Here's how the part is built. I have some questions about the finished solid (model axes, mm). Face numbers are marked on the shaded views. A direction names the side the tool comes from. Round coordinates to 2 decimals unless told otherwise and drop trailing zeros. Write each loop counter-clockwise with the first axis right and the second up, starting at its lowest first coordinate (ties: lowest second). Pieces come first, ordered by that corner, then holes. Notation, with made-up numbers: (47.25, 73) -> (102.25, 73) arc R20 ccw to (102.25, 111) -> close; hole circle Ø3 at (46.5, 12). An arc over 180 degrees is marked (long way). Answer in a Markdown table with one row per item.
from build123d import *

# Parameters (mm, degrees)
SKETCH1_W           = 300
SKETCH1_H           = 56
BOSS_EXTRUDE1_DEPTH = 56
FILLET1_R           = 5
SKETCH2_R           = 27
SKETCH2_W           = 42
SKETCH2_H           = 2
SKETCH2_W_2         = 5
SKETCH2_H_2         = 5
CUT_EXTRUDE1_DEPTH  = 50
SKETCH3_W           = 69.790407192
SKETCH3_H           = 41
CUT_EXTRUDE2_DEPTH  = 25


with BuildPart() as part:
    # Sketch1 → Boss-Extrude1 (new body)
    with BuildSketch(Plane.XY):
        Rectangle(SKETCH1_W, SKETCH1_H)
    extrude(amount=BOSS_EXTRUDE1_DEPTH)

    # Fillet1
    fillet1_edges = [part.edges().sort_by_distance(p)[0] for p in [
        (-150, 0, 0),
        (0, 28, 0),
        (150, 0, 0),
        (-150, 28, 28),
        (150, 28, 28),
    ]]
    fillet(fillet1_edges, radius=FILLET1_R)

    # Sketch2 → Cut-Extrude1 (cut)
    with BuildSketch(Plane.XY.offset(56)):
        with Locations((-71.095356244, 0)):
            Circle(SKETCH2_R)
        with Locations((72.182261243, 0)):
            Rectangle(SKETCH2_W, SKETCH2_H)
        with Locations((110.682261243, 0)):
            Rectangle(SKETCH2_W_2, SKETCH2_H_2)
    extrude(amount=-CUT_EXTRUDE1_DEPTH, mode=Mode.SUBTRACT)

    # Sketch3 → Cut-Extrude2 (cut)
    with BuildSketch(Plane(origin=(0, 28, 0), x_dir=(1, 0, 0), z_dir=(0, 1, 0))):
        with Locations((80.104796404, -30.5)):
            Rectangle(SKETCH3_W, SKETCH3_H)
    extrude(amount=-CUT_EXTRUDE2_DEPTH, mode=Mode.SUBTRACT)


solid = part.part
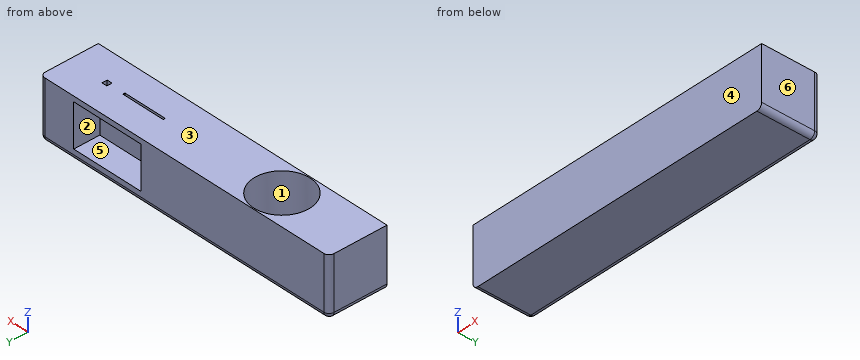
1) I want a section at C-C, the plane x = -92. List the corners of the cut face in (y, z) for me, and give its area (3 significant figures).
Response:
| item | result |
|---|---|
| outline | (-28, 0) -> (23, 0) arc R5 ccw to (28, 5) -> (28, 56) -> (17.09, 56) -> (17.09, 6) -> (-17.09, 6) -> (-17.09, 56) -> (-28, 56) -> close |
| area | 1,420 mm^2 |
2) We'd pull the mould along X, two halves only. Please class the marked faces 4, 5 and 6: +X half, -X half, draft (parallel to the pull), parting line (faces both ways), or undercut.
Response:
| item | result |
|---|---|
| face 4 | draft |
| face 5 | undercut |
| face 6 | +X half |
3) I want a section at D-D, the plane y = 7. List the corners of the cut face in (x, z) for me, and give its area (3 significant figures).
Response:
| item | result |
|---|---|
| outline | (-150, 5) arc R5 ccw to (-145, 0) -> (145, 0) arc R5 ccw to (150, 5) -> (150, 56) -> (-45.02, 56) -> (-45.02, 6) -> (-97.17, 6) -> (-97.17, 56) -> (-150, 56) -> close; hole (45.21, 10) -> (115, 10) -> (115, 51) -> (45.21, 51) -> close |
| area | 11,300 mm^2 |
4) I need wall thicknesses on line 1 (Y direction, x = 61.5, z = 47); line 2 (Z direction, x = -58, y = -15.5); line 3 (Y direction, x = -78, z = 53). Which ranges of each line are inside material? Lowest first, please. Write a range as [from, to].
Response:
| item | result |
|---|---|
| line 1 | y = [-28, -1], [1, 3] |
| line 2 | z = [0, 6] |
| line 3 | y = [-28, -26.1], [26.1, 28] |
5) I want a section at B-B, the plane y = -11. List the corners of the cut face in (x, z) for me, and give its area (3 significant figures).
Response:
| item | result |
|---|---|
| outline | (-150, 5) arc R5 ccw to (-145, 0) -> (145, 0) arc R5 ccw to (150, 5) -> (150, 56) -> (-46.44, 56) -> (-46.44, 6) -> (-95.75, 6) -> (-95.75, 56) -> (-150, 56) -> close |
| area | 14,300 mm^2 |
6) I want a section at A-A, the plane z = 53.5. List the corners of the cut face in (x, y) for me, and give its area (3 significant figures).
Response:
| item | result |
|---|---|
| outline | (-150, -28) -> (150, -28) -> (150, 23) arc R5 ccw to (145, 28) -> (-145, 28) arc R5 ccw to (-150, 23) -> close; hole circle Ø54 at (-71.1, 0); hole (51.18, -1) -> (93.18, -1) -> (93.18, 1) -> (51.18, 1) -> close; hole (108.18, -2.5) -> (113.18, -2.5) -> (113.18, 2.5) -> (108.18, 2.5) -> close |
| area | 14,400 mm^2 |
7) Which directions (+Z, -Z, +X, -X, +Y, -Y) give clear straight access to the entire face, cutting with the end or side of a thin tool? Please do the marked faces 1, 2 and 3.
Response:
| item | result |
|---|---|
| face 1 | +Z |
| face 2 | +Y |
| face 3 | +Z, +X, -X, +Y, -Y |
8) For pin 1 (20.5 mm diameter, centred on x = 70.5, z = 21.5, fed in from +Y), with a flat end and sliding along its axis, tell me the tip position at first contact or that it passes through.
Response:
| item | result |
|---|---|
| pin 1 | stops at y = 3 |
